from build123d import *

# Parameters (mm, degrees)
F0_R     = 6
F0_R_2   = 2.65
F1_DEPTH = 5
F2_R     = 2.65
F3_DEPTH = 25
F4_R     = 4
F4_R_2   = 2.65
F5_DEPTH = 2.5


with BuildPart() as f1:
    # F0 (on Top) → F1 (new body)
    with BuildSketch(Plane.XY):
        Circle(F0_R)
        Circle(F0_R_2, mode=Mode.SUBTRACT)
        Circle(F0_R_2)
    extrude(amount=F1_DEPTH)

    # F2 (on face) → F3 (cut)
    with BuildSketch(Plane(origin=(0, 0, 0), x_dir=(1, 0, 0), z_dir=(0, 0, -1))):
        Circle(F2_R)
    extrude(amount=-F3_DEPTH, mode=Mode.SUBTRACT)

    # F4 (on face) → F5 (cut)
    with BuildSketch(Plane.XY.offset(5)):
        Circle(F4_R)
        Circle(F4_R_2, mode=Mode.SUBTRACT)
    extrude(amount=-F5_DEPTH, mode=Mode.SUBTRACT)


solid = f1.part
Check sheet for the modelled part. Datum: model origin and axes. Units: mm. A direction names the side the tool comes from. Round coordinates to 2 decimals unless told otherwise and drop trailing zeros. Order: outer loops, then holes, each group sorted by start corner. A loop starts at its lowest first (then second) coordinate and runs counter-clockwise, first axis right, second up.
(1) Cross-section at A-A, the plane y = 0. Enter the section's corners in (x, z), and give its area (4 significant figures).
(2) Go/stop test with flat-tipped pins: P1, Ø4, axis at x = 2, y = -3, coming from the +Z side; P2, Ø2, axis at x = 4.5, z = 2, coming from the +Y side. Record where each tip stops, or that it passes through.
(3) Access from +Z, -Z, +X, -X, +Y, -Y to the whole of each face (thin tool, end or side, straight path). Record for faces 4 (the flat face through (3, -1, 2.5)), 5 (the flat face through (-1.42, -3.92, 5)).
(4) Draft check along Y on faces 1 (the flat face through (3, -1, 0)), 2 (the cylindrical face through (2.45, 1.01, 1.23)), 3 (the cylindrical face through (-6, 0, 2)). Enter one of: pulls with the +Y half, pulls with the -Y half, needs draft (parallel to the pull), parting line crosses it, or undercut.
(5) Cross-section at C-C, the plane z = 4.75. Enter the section's corners in (x, y), and give its area (3 significant figures).
(6) Cross-section at D-D, the plane x = -3.5. Enter the section's corners in (y, z).
(7) Scan lines: probe 1 along Y at (x, z) = (0, 4); probe 2 along Y at (x, z) = (0, 1.6); probe 3 along Z at (x, y) = (-3.5, 0.5). Record each from-to range of solid material in increasing order.
Check sheet entries:
1. outline: (-6, 0) - (-2.65, 0) - (-2.65, 2.5) - (-4, 2.5) - (-4, 5) - (-6, 5) - close; (2.65, 0) - (6, 0) - (6, 5) - (4, 5) - (4, 2.5) - (2.65, 2.5) - close
1. area: 26.75 mm2
2. P1: stops at z = 5
2. P2: stops at y = 4.87
3. face 4: +Z
3. face 5: +Z, +X, -X, +Y, -Y
4. face 1: needs draft
4. face 2: undercut
4. face 3: parting line crosses it
5. outline: circle Ø12 at (0, 0); hole circle Ø8 at (0, 0)
5. area: 62.8 mm2
6. outline: (-4.87, 0) - (4.87, 0) - (4.87, 5) - (1.94, 5) - (1.94, 2.5) - (-1.94, 2.5) - (-1.94, 5) - (-4.87, 5) - close
7. probe 1: y = -6 to -4, 4 to 6
7. probe 2: y = -6 to -2.65, 2.65 to 6
7. probe 3: z = 0 to 2.5
